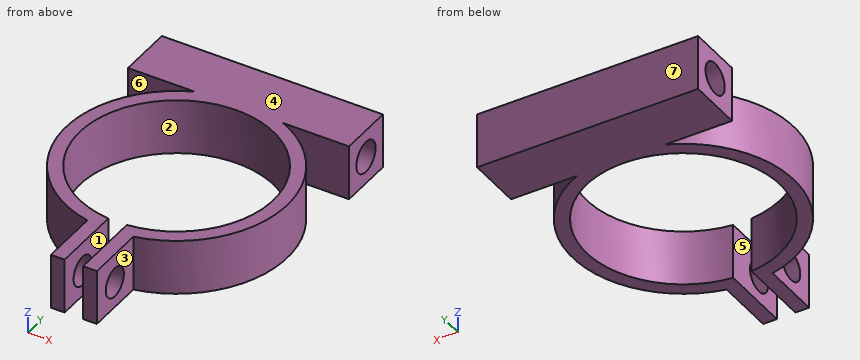
```python
from build123d import *

# Parameters (mm, degrees)
SALIENTE_EXTRUIR1_DEPTH      = 6
TALADRO_DE_MARGEN_PARA_M31_D = 3.4
TALADRO_DE_MARGEN_PARA_M32_D = 3.2


with BuildPart() as part:
    # Croquis1 → Saliente-Extruir1 (new body)
    with BuildSketch(Plane.XY):
        with BuildLine():
            Line((11.975508884, 11), (11.975508884, 17))
            Line((11.975508884, 17), (-12.024491116, 17))
            Line((-12.024491116, 17), (-12.024491116, 11))
            Line((-12.024491116, 11), (-4.795831523, 11))
            ThreePointArc((-4.795831523, 11), (-11.939288491, -1.205566393), (-2.5, -11.736694594))
            Line((-2.5, -11.736694594), (-2.5, -18.20187424))
            Line((-2.5, -18.20187424), (-1, -18.20187424))
            Line((-1, -18.20187424), (-1, -10.45227248))
            ThreePointArc((-1, -10.45227248), (0, 10.5), (1, -10.45227248))
            Line((1, -10.45227248), (1, -18.20187424))
            Line((1, -18.20187424), (2.5, -18.20187424))
            Line((2.5, -18.20187424), (2.5, -11.736694594))
            ThreePointArc((2.5, -11.736694594), (11.939288491, -1.205566393), (4.795831523, 11))
            Line((4.795831523, 11), (11.975508884, 11))
        make_face()
    extrude(amount=SALIENTE_EXTRUIR1_DEPTH)

    # Taladro de margen para M31 (through all)
    with Locations(Plane(origin=(11.975508884, 0, 0), x_dir=(0, 0, -1), z_dir=(1, 0, 0))):
        with Locations((-3, 14)):
            Hole(TALADRO_DE_MARGEN_PARA_M31_D / 2)

    # Taladro de margen para M32 (through all)
    with Locations(Plane.ZY.offset(2.5)):
        with Locations((2.820532603, -15.023895907)):
            Hole(TALADRO_DE_MARGEN_PARA_M32_D / 2)


solid = part.part
```
Can you work these out from the model? Positions are in its coordinate system, mm. Face numbers are marked on the shaded views. A direction names the side the tool comes from. Round coordinates to 2 decimals unless told otherwise and drop trailing zeros. Loops run counter-clockwise (first coordinate to the right, second up) from the corner with the lowest first, then second, coordinate; pieces in that order, holes last. Notation, with made-up numbers: (27.25, 33.25) -> (48.25, 33.25) arc R30 ccw to (48.25, 64.25) -> close; hole circle Ø2 at (72.25, 2). An arc over 180 degrees is marked (long way). One line per item, written item: value. Start each with the question number.
1. If we section it at A-A, the plane y = 14: Write out the boundary of the cut face in (x, z), then the cut area to 3 significant figures.
2. If we mould it in two halves opening along X, with no side actions, what happens to the marked faces 1, 2, 3 and 4? For each: pulls with the +X half, pulls with the -X half, needs draft (parallel to the pull), parting line crosses it, or undercut.
3. If I drill on probe 1 along X at (y, z) = (-11, 4.2); probe 2 along Y at (x, z) = (-9.5, 0.4); probe 3 along Y at (x, z) = (-9, 0.35), over which ranges is the centre line in solid material (lowest first)?
4. For the marked faces 5, 6 and 7, which set-ups out of +Z, -Z, +X, -X, +Y, -Y let a thin tool reach every point of the face, with its end or its side?
5. For pin 1 (1.8 mm diameter, centred on y = -16, z = 2.5, fed in from -X); pin 2 (2 mm diameter, centred on y = 9, z = 2, fed in from -X); pin 3 (3 mm diameter, centred on y = 15, z = 2.5, fed in from +X), each with a flat end and sliding along its axis, tell me the tip position at first contact or that it passes through.
6. If we section it at C-C, the plane x = -9.75: Write out the boundary of the cut face in (y, z), then the cut area to 3 significant figures.
7. If we section it at D-D, the plane z = 3.5: Write out the boundary of the cut face in (x, y), then the cut area to 3 significant figures.
8. If we section it at B-B, the plane x = 1.5: Write out the boundary of the cut face in (y, z), then the cut area to 3 significant figures.
Calculated:
1. outline: (-12.02, 0) -> (11.98, 0) -> (11.98, 1.3) -> (-12.02, 1.3) -> close; (-12.02, 4.7) -> (11.98, 4.7) -> (11.98, 6) -> (-12.02, 6) -> close
1. area: 62.4 mm²
2. face 1: undercut
2. face 2: undercut
2. face 3: pulls with the +X half
2. face 4: needs draft
3. probe 1: x = -4.8 to -1, 1 to 4.8
3. probe 2: y = -7.33 to -4.47, 4.47 to 7.33, 11 to 17
3. probe 3: y = -7.94 to -5.41, 5.41 to 7.94, 11 to 17
4. face 5: +Z, -Z, -Y
4. face 6: +Z, -Z, -X
4. face 7: +Z, -Z, +X, -X, +Y
5. pin 1: stops at x = -2.5
5. pin 2: stops at x = -8.94
5. pin 3: stops at x = 11.98
6. outline: (-7, 0) -> (-3.9, 0) -> (-3.9, 6) -> (-7, 6) -> close; (3.9, 0) -> (7, 0) -> (7, 6) -> (3.9, 6) -> close; (11, 0) -> (17, 0) -> (17, 6) -> (11, 6) -> close; hole circle Ø3.4 at (14, 3)
6. area: 64.1 mm²
7. outline: (-12.02, 11) -> (-4.8, 11) arc R12 ccw to (-2.5, -11.74) -> (-2.5, -13.58) -> (-1, -13.58) -> (-1, -10.45) arc R10.5 cw (long way) to (1, -10.45) -> (1, -13.58) -> (2.5, -13.58) -> (2.5, -11.74) arc R12 ccw to (4.8, 11) -> (11.98, 11) -> (11.98, 12.38) -> (-12.02, 12.38) -> close; (-12.02, 15.62) -> (11.98, 15.62) -> (11.98, 17) -> (-12.02, 17) -> close; (-2.5, -18.2) -> (-1, -18.2) -> (-1, -16.47) -> (-2.5, -16.47) -> close; (1, -18.2) -> (2.5, -18.2) -> (2.5, -16.47) -> (1, -16.47) -> close
7. area: 173 mm²
8. outline: (-18.2, 0) -> (-10.39, 0) -> (-10.39, 6) -> (-18.2, 6) -> close; (10.39, 0) -> (17, 0) -> (17, 6) -> (10.39, 6) -> close; hole circle Ø3.2 at (-15.02, 2.82); hole circle Ø3.4 at (14, 3)
8. area: 69.4 mm²
